CAD build for the part. Positions are in the model's coordinates, mm. A direction names the side the tool comes from. Give positions to 0.01 mm unless a question says otherwise; leave off trailing zeros. Write each loop counter-clockwise with the first axis right and the second up, starting at its lowest first coordinate (ties: lowest second). Pieces come first, ordered by that corner, then holes. Notation, with made-up numbers: (3, 85) - (41, 85) arc R13 ccw to (41, 100) - close; hole circle Ø9 at (71, -14.75). An arc over 180 degrees is marked (long way). Put each result on its own line as item: value. Start each with the question number.
1. Wall check: line 1 (X direction, y = 3.5, z = 28); line 2 (Y direction, x = 2, z = 47.5). Give the ranges that are in metal, low to high.
2. Drop flat-ended pins along their axis: pin 1 (2 mm diameter, centred on x = 2, y = 4, fed in from -Z); pin 2 (2 mm diameter, centred on x = 4, z = 48, fed in from -Y); pin 3 (2 mm diameter, centred on y = 11.5, z = 51.5, fed in from -X). Give the stop position or say it passes through.
3. Cut at B-B on z = 17. List the corners of the cut face in (x, y).
4. Tool access for faces 5 (the flat face through (8, 22, 32)), 6 (the flat face through (0, 10, 32)): list every direction of +Z, -Z, +X, -X, +Y, -Y with a clear straight run to the whole face (end or side of a thin tool).
5. Cut at D-D on x = 1.25. List the corners of the cut face in (y, z), and give its area (3 significant figures).
6. Cut at A-A on y = 13. List the corners of the cut face in (x, z).
7. Cut at C-C on z = 22. List the corners of the cut face in (x, y), and give its area (3 significant figures).
8. Mould opens along Z. For faces 1 (the cylindrical face through (0.254, 15.285, 47.168)), 2 (the flat face through (0.3, 9.9, 56.934)), 3 (the flat face through (8, 22.5, 32)), 4 (the cylindrical face through (0.25, 15.02, 15.97)) say: +Z half, -Z half, draft (parallel to the pull), parting line (faces both ways), or undercut.
from build123d import *

# Parameters (mm, degrees)
SKETCH_1_W                  = 50
SKETCH_1_H                  = 25
EXTRUDE_1_DEPTH             = 0.5
SKETCH_2_W                  = 50
SKETCH_2_H                  = 0.5
EXTRUDE_2_DEPTH             = 15
HOLE_WIZARD_3_6_3_6_1_D     = 3.6
HOLE_WIZARD_3_6_3_6_1_DEPTH = 10
HOLE_WIZARD_3_6_3_6_1_TIP   = 1.081549114


with BuildPart() as part:
    # Эскиз1 → Бобышка-Вытянуть1 (new body)
    with BuildSketch(Plane(origin=(0, 0, 0), x_dir=(0, 0, -1), z_dir=(1, 0, 0))):
        with Locations((-31.933808614, 10.000042269)):
            Rectangle(SKETCH_1_W, SKETCH_1_H)
    extrude(amount=EXTRUDE_1_DEPTH)

    # Эскиз2 → Бобышка-Вытянуть2 (add)
    with BuildSketch(Plane(origin=(0.5, 0, 0), x_dir=(0, 0, -1), z_dir=(1, 0, 0))):
        with Locations((-31.933808614, 22.250042269)):
            Rectangle(SKETCH_2_W, SKETCH_2_H)
    extrude(amount=EXTRUDE_2_DEPTH)

    # Диаметр отверстия Ø3.6 (3.6)1
    with Locations(Plane.ZY):
        with Locations((16.933808614, 13.500042269), (46.933808614, 13.500042269)):
            Hole(HOLE_WIZARD_3_6_3_6_1_D / 2, depth=HOLE_WIZARD_3_6_3_6_1_DEPTH)
            with Locations((0, 0, -(HOLE_WIZARD_3_6_3_6_1_DEPTH + HOLE_WIZARD_3_6_3_6_1_TIP / 2))):  # 118° drill point
                Cone(0, HOLE_WIZARD_3_6_3_6_1_D / 2, HOLE_WIZARD_3_6_3_6_1_TIP, mode=Mode.SUBTRACT)


solid = part.part
Report:
1. line 1: x = 0 to 0.5
1. line 2: y = 22 to 22.5
2. pin 1: passes through
2. pin 2: stops at y = 22
2. pin 3: stops at x = 0
3. outline: (0, -2.5) - (0.5, -2.5) - (0.5, 11.7) - (0, 11.7) - close; (0, 15.3) - (0.5, 15.3) - (0.5, 22) - (15.5, 22) - (15.5, 22.5) - (0, 22.5) - close
4. face 5: +Z, -Z, +X, -Y
4. face 6: +Z, -Z, -X, +Y, -Y
5. outline: (22, 6.93) - (22.5, 6.93) - (22.5, 56.93) - (22, 56.93) - close
5. area: 25.0 mm²
6. outline: (0, 6.93) - (0.5, 6.93) - (0.5, 15.2) - (0, 15.2) - close; (0, 18.66) - (0.5, 18.66) - (0.5, 45.2) - (0, 45.2) - close; (0, 48.66) - (0.5, 48.66) - (0.5, 56.93) - (0, 56.93) - close
7. outline: (0, -2.5) - (0.5, -2.5) - (0.5, 22) - (15.5, 22) - (15.5, 22.5) - (0, 22.5) - close
7. area: 20.0 mm²
8. face 1: undercut
8. face 2: +Z half
8. face 3: draft
8. face 4: undercut
